Answer from the drawing. Dimensions are ordinates in mm from the lowest x, y and z of the part. Round coordinates to 2 decimals unless told otherwise and drop trailing zeros. Loops run counter-clockwise (first coordinate to the right, second up) from the corner with the lowest first, then second, coordinate; pieces in that order, holes last. Notation, with made-up numbers: (51.5, 40.5) - (74.5, 40.5) arc R24 cw to (74.5, 69.5) - close; hole circle Ø6 at (-30.5, -20). An arc over 180 degrees is marked (long way). Answer as CSV lines item,"result".
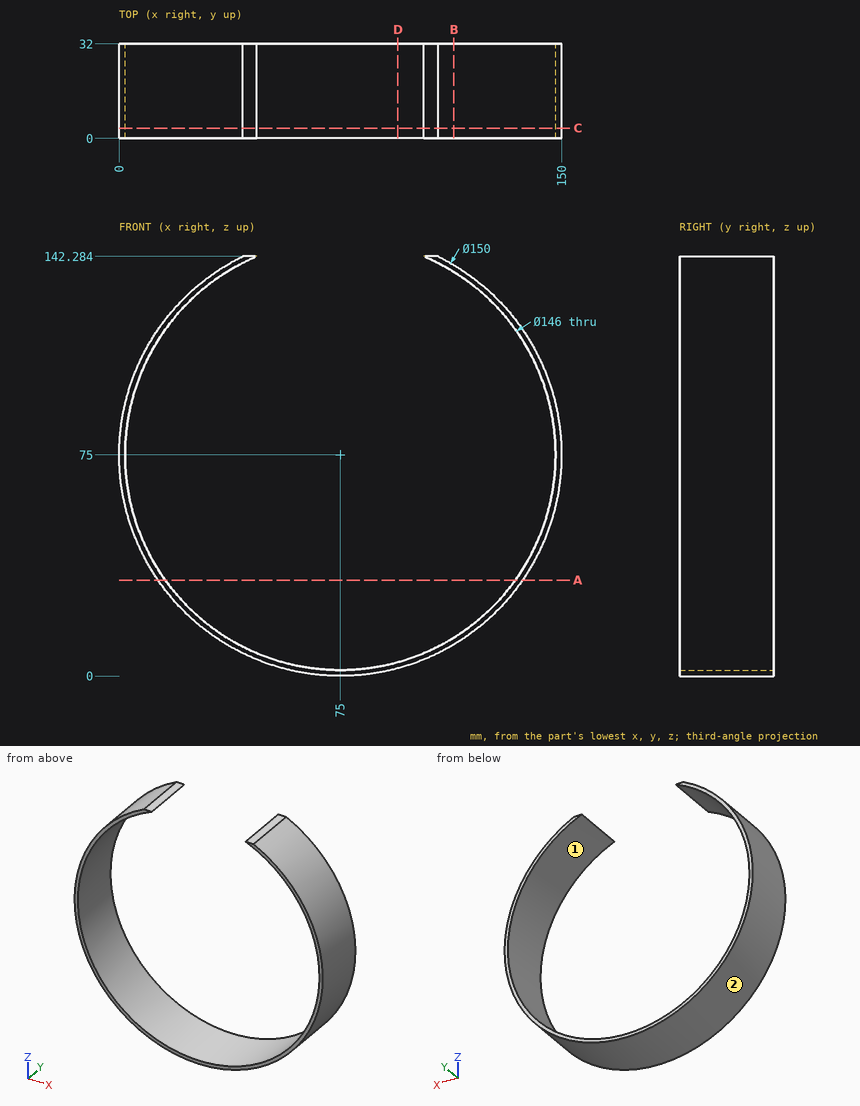
1) A cutting plane is placed at D-D, the plane x = 94.5. Determine the outline of the cut face in (y, z).
Entries:
outline,"(0, 2.58) - (32, 2.58) - (32, 4.65) - (0, 4.65) - close"
2) A cutting plane is placed at C-C, the plane y = 3.5. Determine the outline of the cut face in (x, z).
Entries:
outline,"(41.87, 142.28) arc R75 ccw (long way) to (108.13, 142.28) - (103.32, 142.28) arc R73 cw (long way) to (46.68, 142.28) - close"
3) Find the intervals of material crossed by line 1 (Z direction, x = 38, y = 16.5); line 2 (X direction, y = 8, z = 83); line 3 (X direction, y = 17.5, z = 86.5), in increasing order.
Entries:
line 1,"z = 9.76 to 12.07, 137.93 to 140.24"
line 2,"x = 0.43 to 2.44, 147.56 to 149.57"
line 3,"x = 0.89 to 2.91, 147.09 to 149.11"
4) A cutting plane is placed at B-B, the plane x = 113.5. Determine the outline of the cut face in (y, z).
Entries:
outline,"(0, 10.64) - (32, 10.64) - (32, 12.98) - (0, 12.98) - close; (0, 137.02) - (32, 137.02) - (32, 139.36) - (0, 139.36) - close"
5) The mould has two halves that part along Z. Classify the marked faces 1 and 2: pulls with the +Z half, pulls with the -Z half, needs draft (parallel to the pull), parting line crosses it, or undercut.
Entries:
face 1,"undercut"
face 2,"parting line crosses it"
6) A cutting plane is placed at A-A, the plane z = 32.5. Determine the outline of the cut face in (x, y).
Entries:
outline,"(13.2, 0) - (15.65, 0) - (15.65, 32) - (13.2, 32) - close; (134.35, 0) - (136.8, 0) - (136.8, 32) - (134.35, 32) - close"
7) Each of these flat-tipped pins is pushed along its axis until it touches: P1, Ø1.5, axis at x = 133, y = 23, coming from the -Z side; P2, Ø1.5, axis at y = 11, z = 100, coming from the +X side; P3, Ø2, axis at y = 14, z = 78, coming from the +X side. Where does it stop, or does it pass through?
Entries:
P1,"stops at z = 26.55"
P2,"stops at x = 145.97"
P3,"stops at x = 149.97"
